```python
from build123d import *

# Parameters (mm, degrees)
F0_W        = 40
F0_H        = 26.199
F0_W_2      = 10
F0_H_2      = 10
F1_DEPTH    = 2
F2_T1_DEPTH = 56.5285930149


# Not quite as in the source:
# - a fillet or chamfer that OpenCascade refuses, or shapes differently, is made with other operations: its cross-section is extruded or revolved along the edge and cut away or added


with BuildPart() as f1:
    # F0 (on Right) → F1 (new body)
    with BuildSketch(Plane.YZ):
        Rectangle(F0_W, F0_H)
        with Locations((-12, 5.0995)):
            Rectangle(F0_W_2, F0_H_2, mode=Mode.SUBTRACT)
        with Locations((12, 5.0995)):
            Rectangle(F0_W_2, F0_H_2, mode=Mode.SUBTRACT)
    extrude(amount=F1_DEPTH)

    # F2: chamfer of 2.16713 x 3.199 on 1 edges, made by hand

    # F2_s2 → F2_t1 (cut)
    with BuildSketch(Plane.XZ.offset(-28.2642965075)):
        Polygon((2.16713, 13.0995), (0, 9.9005), (0, 13.0995), align=None)
    extrude(amount=F2_T1_DEPTH, mode=Mode.SUBTRACT)


solid = f1.part
```
Can you work these out from the model? Positions are in its coordinate system, mm. A direction names the side the tool comes from. Give positions to 0.01 mm unless a question says otherwise; leave off trailing zeros. Write each loop counter-clockwise with the first axis right and the second up, starting at its lowest first coordinate (ties: lowest second). Pieces come first, ordered by that corner, then holes. Notation, with made-up numbers: (78, 18.5) -> (94, 18.5) arc R28 cw to (94, 55.5) -> close; hole circle Ø7 at (-10, -16.5). An arc over 180 degrees is marked (long way). Write item = value, one per line.
(1) I need wall thicknesses on probe 1 along Y at (x, z) = (1.1, 2.25); probe 2 along Z at (x, y) = (1.3, 15.5); probe 3 along Z at (x, y) = (1.95, -12). Which ranges of each line are inside material? Lowest first, please. Write a range as from..to.
Worked out:
probe_1 = -20..-17, -7..7, 17..20
probe_2 = -13.1..0.1, 10.1..11.82
probe_3 = -13.1..0.1, 10.1..12.78
(2) I'm going to push a flat-ended pin straight in: P1, Ø0.6, axis at x = 0.5, y = 14, coming from the +Z side. Where does the tip first touch, or does it pass through?
Worked out:
P1 = 11.08
(3) Suppose I cut it at A-A on z = 2.5. Write out the boundary of the cut face in (x, y).
Worked out:
outline = (0, -20) -> (2, -20) -> (2, -17) -> (0, -17) -> close; (0, -7) -> (2, -7) -> (2, 7) -> (0, 7) -> close; (0, 17) -> (2, 17) -> (2, 20) -> (0, 20) -> close
(4) For faces 5 (the face through (1.014, 0.28, 11.397)), 6 (the face through (1, -7, 5)), which set-ups out of +Z, -Z, +X, -X, +Y, -Y let a thin tool reach every point of the face, with its end or its side?
Worked out:
face_5 = +Z, -X, +Y, -Y
face_6 = +X, -X
(5) Suppose I cut it at C-C on x = 1. Write out the boundary of the cut face in (y, z).
Worked out:
outline = (-20, -13.1) -> (20, -13.1) -> (20, 11.38) -> (-20, 11.38) -> close; hole (-17, 0.1) -> (-7, 0.1) -> (-7, 10.1) -> (-17, 10.1) -> close; hole (7, 0.1) -> (17, 0.1) -> (17, 10.1) -> (7, 10.1) -> close
(6) Thinking about a two-plate mould opening in Y: for faces 1 (the face through (1, -20, 0)), 2 (the face through (1, -12, 0.099)), 3 (the face through (1, 20, 0)), 4 (the face through (2, 0, 0)), which applies, released by +Y, released by -Y, zero draft, split by the parting line, or undercut?
Worked out:
face_1 = released by -Y
face_2 = undercut
face_3 = released by +Y
face_4 = zero draft
(7) Suppose I cut it at D-D on y = -4. Write out the boundary of the cut face in (x, z), then the cut area to 3 significant figures.
Worked out:
outline = (0, -13.1) -> (2, -13.1) -> (2, 12.85) -> (0, 9.9) -> close
area = 49.0 mm^2
(8) Suppose I cut it at B-B on y = -9. Write out the boundary of the cut face in (x, z).
Worked out:
outline = (0, -13.1) -> (2, -13.1) -> (2, 0.1) -> (0, 0.1) -> close; (0.13, 10.1) -> (2, 10.1) -> (2, 12.85) -> close
